```python
from build123d import *

# Parameters (mm, degrees)
F0_W     = 500
F0_H     = 75
F1_DEPTH = 6.35
F2_W     = 50
F2_H     = 6.35
F3_DEPTH = 6.35
F4_W     = 6.35
F4_H     = 10
F5_DEPTH = 6.351
F6_R     = 6.35
F7_DEPTH = 25


# Not quite as in the source:
# - a length typed as a fraction of an inch, garbled in the dataset ("3 / 203.2 mm" for 3/8 in), is restored


with BuildPart() as f1:
    # F0 (on Top) → F1 (new body)
    with BuildSketch(Plane.XY):
        Rectangle(F0_W, F0_H)
    extrude(amount=F1_DEPTH)

    # F2 (on face) → F3 (join, through all)
    with BuildSketch(Plane.XY.offset(6.35)):
        with Locations((-200, -40.675)):
            Rectangle(F2_W, F2_H)
        with Locations((-100, -40.675)):
            Rectangle(F2_W, F2_H)
        with Locations((0, -40.675)):
            Rectangle(F2_W, F2_H)
        with Locations((100, -40.675)):
            Rectangle(F2_W, F2_H)
        with Locations((200, -40.675)):
            Rectangle(F2_W, F2_H)
    extrude(amount=-F3_DEPTH)

    # F4 (on face) → F5 (cut, through all)
    with BuildSketch(Plane.XY.offset(6.35)):
        with Locations((246.825, 22.5)):
            Rectangle(F4_W, F4_H)
        with Locations((246.825, 0)):
            Rectangle(F4_W, F4_H)
        with Locations((246.825, -22.5)):
            Rectangle(F4_W, F4_H)
        with Locations((-246.825, 22.5)):
            Rectangle(F4_W, F4_H)
        with Locations((-246.825, 0)):
            Rectangle(F4_W, F4_H)
        with Locations((-246.825, -22.5)):
            Rectangle(F4_W, F4_H)
    extrude(amount=-F5_DEPTH, mode=Mode.SUBTRACT)

    # F6 (on face) → F7 (cut)
    with BuildSketch(Plane.XY.offset(6.35)):
        with Locations((-200, 17.5)):
            Circle(F6_R)
        with Locations((-120, 17.5)):
            Circle(F6_R)
        with Locations((-40, 17.5)):
            Circle(F6_R)
        with Locations((40, 17.5)):
            Circle(F6_R)
        with Locations((120, 17.5)):
            Circle(F6_R)
        with Locations((200, 17.5)):
            Circle(F6_R)
    extrude(amount=-F7_DEPTH, mode=Mode.SUBTRACT)


solid = f1.part
```
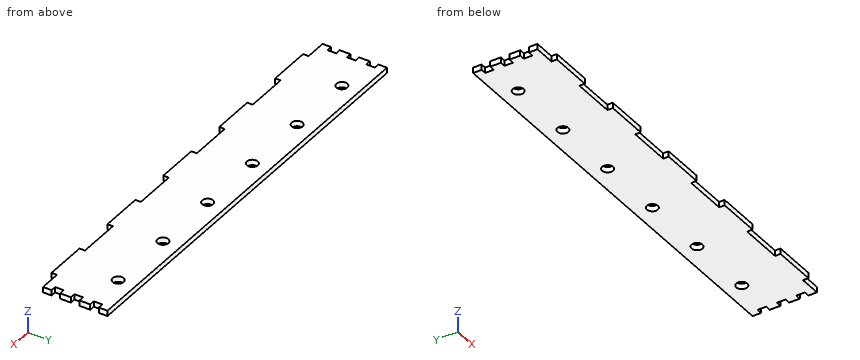
Work out the finished part from the listing and answer in its coordinate system (mm). Give positions to 0.01 mm unless a question says otherwise; leave off trailing zeros. Loops run counter-clockwise (first coordinate to the right, second up) from the corner with the lowest first, then second, coordinate; pieces in that order, holes last. Notation, with made-up numbers: (-33, 26) - (-18, 26) arc R31 ccw to (-18, 54) - close; hole circle Ø2 at (-28, -23). An arc over 180 degrees is marked (long way). Use CSV: the item, a comma, the result in double quotes. Start each with the question number.
(1) Find section B-B, the plane z = 3.75. Count the separate pieces of the cut face and the enclosed holes in it, plus the area to 3 significant figures.
(2) Find section A-A, the plane x = -40. Determine the outline of the cut face in (y, z), plus the area to 3 significant figures.
(3) Find section C-C, the plane x = -120. Determine the outline of the cut face in (y, z), plus the area to 3 significant figures.
(4) Find the intervals of material crossed by L1, parallel to Y at x = 40, z = 2; L2, parallel to Y at x = 27, z = 0.5; L3, parallel to Y at x = 200, z = 4.5, in increasing order.
(5) Each of these flat-tipped pins is pushed along its axis until it touches: pin 1 (3 mm diameter, centred on x = 57.5, z = 4, fed in from -Y); pin 2 (1.9 mm diameter, centred on y = -25, z = 4.5, fed in from +X); pin 3 (3 mm diameter, centred on y = -39.5, z = 3.5, fed in from +X). Where does it stop, or does it pass through?
Results found:
1,separate pieces,"1"
1,enclosed holes,"6"
1,area,"37,900 mm^2"
2,outline,"(-37.5, 0) - (11.15, 0) - (11.15, 6.35) - (-37.5, 6.35) - close; (23.85, 0) - (37.5, 0) - (37.5, 6.35) - (23.85, 6.35) - close"
2,area,"396 mm^2"
3,outline,"(-43.85, 0) - (11.15, 0) - (11.15, 6.35) - (-43.85, 6.35) - close; (23.85, 0) - (37.5, 0) - (37.5, 6.35) - (23.85, 6.35) - close"
3,area,"436 mm^2"
4,L1,"-37.5 to 11.15, 23.85 to 37.5"
4,L2,"-37.5 to 37.5"
4,L3,"-43.85 to 11.15, 23.85 to 37.5"
5,pin 1,"y = -37.5"
5,pin 2,"x = 243.65"
5,pin 3,"x = 225"
